```python
from build123d import *

# Parameters (mm, degrees)
F0_W     = 55
F0_H     = 15
F1_DEPTH = 5
F2_W     = 5
F2_H     = 15
F3_DEPTH = 15
F4_R     = 2.5
F5_DEPTH = 25
F6_R     = 2.5
F7_DEPTH = 25
F8_R     = 2.05
F9_DEPTH = 45.001


with BuildPart() as f1:
    # F0 (on Top) → F1 (new body)
    with BuildSketch(Plane.XY):
        with Locations((12.159763, 0.993737)):
            Rectangle(F0_W, F0_H)
    extrude(amount=F1_DEPTH)

    # F2 (on face) → F3 (join)
    with BuildSketch(Plane.XY.offset(5)):
        with Locations((-2.840237, 0.993737)):
            Rectangle(F2_W, F2_H)
        with Locations((27.159763, 0.993737)):
            Rectangle(F2_W, F2_H)
    extrude(amount=F3_DEPTH)

    # F4 (on face) → F5 (cut)
    with BuildSketch(Plane.XY.offset(5)):
        with Locations((-10.340237, 0.993737)):
            Circle(F4_R)
    extrude(amount=-F5_DEPTH, mode=Mode.SUBTRACT)

    # F6 (on face) → F7 (cut)
    with BuildSketch(Plane.XY.offset(5)):
        with Locations((34.659763, 0.993737)):
            Circle(F6_R)
    extrude(amount=-F7_DEPTH, mode=Mode.SUBTRACT)

    # F8 (on face) → F9 (cut, through all)
    with BuildSketch(Plane(origin=(-5.340237, 0, 0), x_dir=(0, -1, 0), z_dir=(-1, 0, 0))):
        with Locations((-0.993737, 13.786643)):
            Circle(F8_R)
    extrude(amount=-F9_DEPTH, mode=Mode.SUBTRACT)


solid = f1.part
```
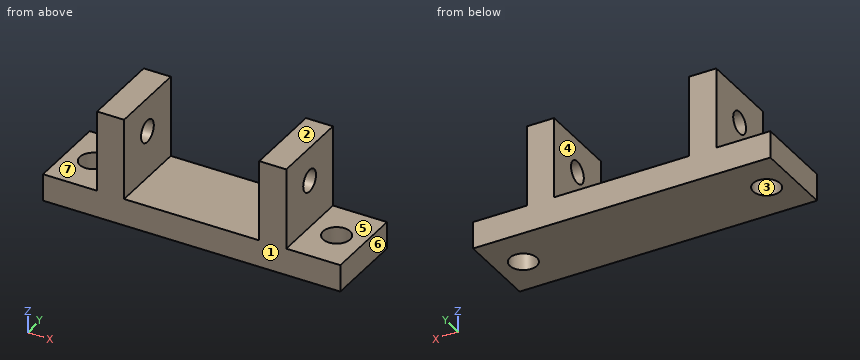
Design review of the part built by this model. Coordinates are the model's own, in mm. Face numbers are marked on the shaded views. A direction names the side the tool comes from. Round coordinates to 2 decimals unless told otherwise and drop trailing zeros. Write each loop counter-clockwise with the first axis right and the second up, starting at its lowest first coordinate (ties: lowest second). Pieces come first, ordered by that corner, then holes. Notation, with made-up numbers: (32, 11) -> (46, 11) arc R22 cw to (46, 25) -> close; hole circle Ø10 at (33, 26). An arc over 180 degrees is marked (long way). Answer in a Markdown table with one row per item.
Q1. Take a section at D-D, the plane z = 13. State the section outline as (x, y) points, then the cut area to 3 significant figures.
The answers:
| item | result |
|---|---|
| outline | (-5.34, -6.51) -> (-0.34, -6.51) -> (-0.34, -0.9) -> (-5.34, -0.9) -> close; (-5.34, 2.89) -> (-0.34, 2.89) -> (-0.34, 8.49) -> (-5.34, 8.49) -> close; (24.66, -6.51) -> (29.66, -6.51) -> (29.66, -0.9) -> (24.66, -0.9) -> close; (24.66, 2.89) -> (29.66, 2.89) -> (29.66, 8.49) -> (24.66, 8.49) -> close |
| area | 112 mm² |
Q2. Draft analysis for pull direction Y (two halves, no side actions). For the marked faces 1, 2 and 3, state which applies: +Y half, -Y half, draft (parallel to the pull), parting line (faces both ways), or undercut.
The answers:
| item | result |
|---|---|
| face 1 | -Y half |
| face 2 | draft |
| face 3 | undercut |
Q3. Clearance check with flat-ended pins moving along their axes: pin 1 Ø6 at (x, y) = (13.5, -3.5) entering from +Z; pin 2 Ø7.5 at (y, z) = (4.5, 15) entering from +X; pin 3 Ø4.5 at (y, z) = (2.5, 12.5) entering from -X. State where each tip first meets the part, or that it passes through.
The answers:
| item | result |
|---|---|
| pin 1 | z = 5 |
| pin 2 | x = 29.66 |
| pin 3 | x = -5.34 |
Q4. Take a section at A-A, the plane y = 0. State the section outline as (x, z) points.
The answers:
| item | result |
|---|---|
| outline | (-15.34, 0) -> (-12.63, 0) -> (-12.63, 5) -> (-15.34, 5) -> close; (-8.05, 0) -> (32.37, 0) -> (32.37, 5) -> (29.66, 5) -> (29.66, 11.99) -> (24.66, 11.99) -> (24.66, 5) -> (-0.34, 5) -> (-0.34, 11.99) -> (-5.34, 11.99) -> (-5.34, 5) -> (-8.05, 5) -> close; (-5.34, 15.58) -> (-0.34, 15.58) -> (-0.34, 20) -> (-5.34, 20) -> close; (24.66, 15.58) -> (29.66, 15.58) -> (29.66, 20) -> (24.66, 20) -> close; (36.95, 0) -> (39.66, 0) -> (39.66, 5) -> (36.95, 5) -> close |
Q5. Take a section at B-B, the plane z = 6.25. State the section outline as (x, y) points.
The answers:
| item | result |
|---|---|
| outline | (-5.34, -6.51) -> (-0.34, -6.51) -> (-0.34, 8.49) -> (-5.34, 8.49) -> close; (24.66, -6.51) -> (29.66, -6.51) -> (29.66, 8.49) -> (24.66, 8.49) -> close |
Q6. Take a section at C-C, the plane y = -4.5. State the section outline as (x, z) points.
The answers:
| item | result |
|---|---|
| outline | (-15.34, 0) -> (39.66, 0) -> (39.66, 5) -> (29.66, 5) -> (29.66, 20) -> (24.66, 20) -> (24.66, 5) -> (-0.34, 5) -> (-0.34, 20) -> (-5.34, 20) -> (-5.34, 5) -> (-15.34, 5) -> close |
Q7. For the marked faces 4, 5, 6 and 7, list the 3-axis set-ups (+Z, -Z, +X, -X, +Y, -Y) from which the entire face can be reached by the end or side of a thin tool; tool diameter is ignored.
The answers:
| item | result |
|---|---|
| face 4 | +Z, +Y, -Y |
| face 5 | +Z, +X, +Y, -Y |
| face 6 | +Z, -Z, +X, +Y, -Y |
| face 7 | +Z, -X, +Y, -Y |
Q8. To check wall thickness, follow L1, parallel to X at y = 1, z = 9.5; L2, parallel to Z at x = 3.5, y = 1; L3, parallel to Z at x = 29, y = 1.5. State the ranges of each line that lie inside material, in increasing order. Write a range as [from, to].
The answers:
| item | result |
|---|---|
| L1 | [-5.34, -0.34], [24.66, 29.66] |
| L2 | [0, 5] |
| L3 | [0, 11.8], [15.77, 20] |
